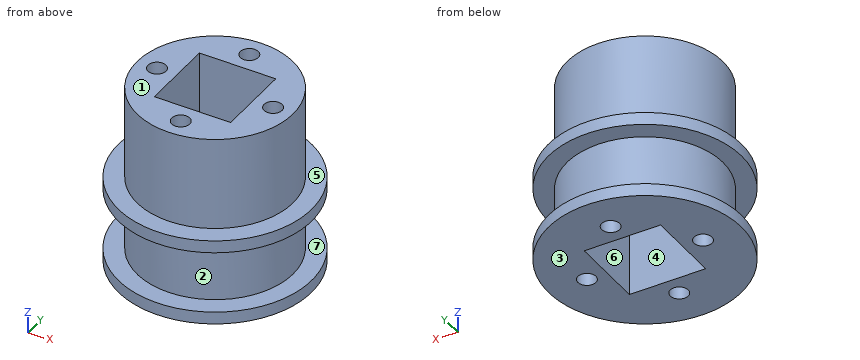
from build123d import *

# Parameters (mm, degrees)
SKETCH1_R           = 12.5
BOSS_EXTRUDE1_DEPTH = 7.5
SKETCH13_R          = 15.5
BOSS_EXTRUDE2_DEPTH = 2
SKETCH14_R          = 12.5
BOSS_EXTRUDE3_DEPTH = 10
SKETCH15_R          = 15.5
BOSS_EXTRUDE4_DEPTH = 2
CUT_EXTRUDE1_REACH  = 38.352
SKETCH8_W           = 12.25
SKETCH8_H           = 12.25
CUT_EXTRUDE4_REACH  = 38.352
SKETCH11_R          = 1.45


with BuildPart() as part:
    # Sketch1 → Boss-Extrude1 (new, symmetric)
    with BuildSketch(Plane.XY):
        Circle(SKETCH1_R)
    extrude(amount=BOSS_EXTRUDE1_DEPTH, both=True)

    # Sketch13 → Boss-Extrude2 (add)
    with BuildSketch(Plane(origin=(0, 0, -7.5), x_dir=(-1, 0, 0), z_dir=(0, 0, -1))):
        Circle(SKETCH13_R)
    extrude(amount=BOSS_EXTRUDE2_DEPTH)

    # Sketch14 → Boss-Extrude3 (add)
    with BuildSketch(Plane(origin=(0, 0, -9.5), x_dir=(-1, 0, 0), z_dir=(0, 0, -1))):
        with Locations(Location((0, 0, 0), (0, 0, 180))):
            Circle(SKETCH14_R)
    extrude(amount=BOSS_EXTRUDE3_DEPTH)

    # Sketch15 → Boss-Extrude4 (add)
    with BuildSketch(Plane(origin=(0, 0, -19.5), x_dir=(-1, 0, 0), z_dir=(0, 0, -1))):
        Circle(SKETCH15_R)
    extrude(amount=BOSS_EXTRUDE4_DEPTH)

    # Sketch8 → Cut-Extrude1 (cut, up to next)
    with BuildSketch(Plane.XY.offset(7.5), mode=Mode.PRIVATE) as cut_extrude1_sk1:
        Rectangle(SKETCH8_W, SKETCH8_H)
    cut_extrude1_tool1 = extrude(cut_extrude1_sk1.sketch, amount=-CUT_EXTRUDE1_REACH, mode=Mode.PRIVATE) & part.part
    add(cut_extrude1_tool1.solids().sort_by_distance((0, 0, 7.5))[0], mode=Mode.SUBTRACT)

    # Sketch11 → Cut-Extrude4 (cut, up to next)
    with BuildSketch(Plane.XY.offset(7.5), mode=Mode.PRIVATE) as cut_extrude4_sk1:
        with Locations((9.315, 0)):
            Circle(SKETCH11_R)
    cut_extrude4_tool1 = extrude(cut_extrude4_sk1.sketch, amount=-CUT_EXTRUDE4_REACH, mode=Mode.PRIVATE) & part.part
    # Sketch11 → Cut-Extrude4 (cut, up to next)
    with BuildSketch(Plane.XY.offset(7.5), mode=Mode.PRIVATE) as cut_extrude4_sk2:
        with Locations((0, -9.315)):
            Circle(SKETCH11_R)
    cut_extrude4_tool2 = extrude(cut_extrude4_sk2.sketch, amount=-CUT_EXTRUDE4_REACH, mode=Mode.PRIVATE) & part.part
    # Sketch11 → Cut-Extrude4 (cut, up to next)
    with BuildSketch(Plane.XY.offset(7.5), mode=Mode.PRIVATE) as cut_extrude4_sk3:
        with Locations((-9.315, 0)):
            Circle(SKETCH11_R)
    cut_extrude4_tool3 = extrude(cut_extrude4_sk3.sketch, amount=-CUT_EXTRUDE4_REACH, mode=Mode.PRIVATE) & part.part
    # Sketch11 → Cut-Extrude4 (cut, up to next)
    with BuildSketch(Plane.XY.offset(7.5), mode=Mode.PRIVATE) as cut_extrude4_sk4:
        with Locations((0, 9.315)):
            Circle(SKETCH11_R)
    cut_extrude4_tool4 = extrude(cut_extrude4_sk4.sketch, amount=-CUT_EXTRUDE4_REACH, mode=Mode.PRIVATE) & part.part
    add(cut_extrude4_tool1.solids().sort_by_distance((9.315, 0, 7.5))[0], mode=Mode.SUBTRACT)
    add(cut_extrude4_tool2.solids().sort_by_distance((0, -9.315, 7.5))[0], mode=Mode.SUBTRACT)
    add(cut_extrude4_tool3.solids().sort_by_distance((-9.315, 0, 7.5))[0], mode=Mode.SUBTRACT)
    add(cut_extrude4_tool4.solids().sort_by_distance((0, 9.315, 7.5))[0], mode=Mode.SUBTRACT)


solid = part.part
Work out the finished part from the listing and answer in its coordinate system (mm). Face numbers are marked on the shaded views. A direction names the side the tool comes from. Round coordinates to 2 decimals unless told otherwise and drop trailing zeros. Loops run counter-clockwise (first coordinate to the right, second up) from the corner with the lowest first, then second, coordinate; pieces in that order, holes last. Notation, with made-up numbers: (7.5, -29.75) -> (53.5, -29.75) arc R23 cw to (53.5, 9.25) -> close; hole circle Ø1 at (15, 77.25). An arc over 180 degrees is marked (long way). Use one line per item in the form item = value.
(1) Find section C-C on z = -5. Give the vertices of the cut face in (x, y) (3 decimals), then the cut area to 3 significant figures.
Answer list:
outline = circle Ø25 at (0, 0); hole circle Ø2.9 at (-9.315, 0); hole (-6.125, -6.125) -> (6.125, -6.125) -> (6.125, 6.125) -> (-6.125, 6.125) -> close; hole circle Ø2.9 at (0, -9.315); hole circle Ø2.9 at (0, 9.315); hole circle Ø2.9 at (9.315, 0)
area = 314 mm2
(2) For a pull along Z with two mould halves and no side action, classify the marked faces 1, 2, 3 and 4 as released by +Z, released by -Z, zero draft, split by the parting line, or undercut.
Answer list:
face_1 = released by +Z
face_2 = undercut
face_3 = released by -Z
face_4 = zero draft
(3) A tool of negligible diameter and unlimited length cuts with its end or side. For the marked faces 5, 6 and 7, from which of +Z, -Z, +X, -X, +Y, -Y can it reach the whole face along a straight path? Write none if from no direction.
Answer list:
face_5 = +Z
face_6 = +Z, -Z
face_7 = none
(4) Flat-ended cylindrical pins translate along their axes: P1, Ø2, axis at x = -12.5, z = -12, coming from the -Y side; P2, Ø2.5, axis at x = -9.315, y = 0, coming from the -Z side; P3, Ø5, axis at x = 1.5, z = 2.5, coming from the -Y side; P4, Ø8, axis at y = -10.5, z = -0.5, coming from the -X side. Find the tip coordinate at first contact, or state that the pin passes through.
Answer list:
P1 = -4.9
P2 = through
P3 = -12.5
P4 = -10.68
(5) Straight lines are drawn through the part: line 1 (Y direction, x = 0, z = -10.75) (3 decimals); line 2 (Z direction, x = -11.5, y = -8.5); line 3 (X direction, y = -0.5, z = -4) (3 decimals). For each, find the intervals that lie inside material, in ascending order.
Answer list:
line_1 = -12.5 to -10.765, -7.865 to -6.125, 6.125 to 7.865, 10.765 to 12.5
line_2 = -21.5 to -19.5, -9.5 to -7.5
line_3 = -12.49 to -10.676, -7.954 to -6.125, 6.125 to 7.954, 10.676 to 12.49
(6) Find section D-D on y = 10. Give the vertices of the cut face in (x, z).
Answer list:
outline = (-11.84, -21.5) -> (-1.28, -21.5) -> (-1.28, 7.5) -> (-7.5, 7.5) -> (-7.5, -7.5) -> (-11.84, -7.5) -> (-11.84, -9.5) -> (-7.5, -9.5) -> (-7.5, -19.5) -> (-11.84, -19.5) -> close; (1.28, -21.5) -> (11.84, -21.5) -> (11.84, -19.5) -> (7.5, -19.5) -> (7.5, -9.5) -> (11.84, -9.5) -> (11.84, -7.5) -> (7.5, -7.5) -> (7.5, 7.5) -> (1.28, 7.5) -> close
(7) Find section A-A on y = 0. Give the vertices of the cut face in (x, z) (3 decimals), then the cut area to 3 significant figures.
Answer list:
outline = (-15.5, -21.5) -> (-10.765, -21.5) -> (-10.765, 7.5) -> (-12.5, 7.5) -> (-12.5, -7.5) -> (-15.5, -7.5) -> (-15.5, -9.5) -> (-12.5, -9.5) -> (-12.5, -19.5) -> (-15.5, -19.5) -> close; (-7.865, -21.5) -> (-6.125, -21.5) -> (-6.125, 7.5) -> (-7.865, 7.5) -> close; (6.125, -21.5) -> (7.865, -21.5) -> (7.865, 7.5) -> (6.125, 7.5) -> close; (10.765, -21.5) -> (15.5, -21.5) -> (15.5, -19.5) -> (12.5, -19.5) -> (12.5, -9.5) -> (15.5, -9.5) -> (15.5, -7.5) -> (12.5, -7.5) -> (12.5, 7.5) -> (10.765, 7.5) -> close
area = 226 mm2
